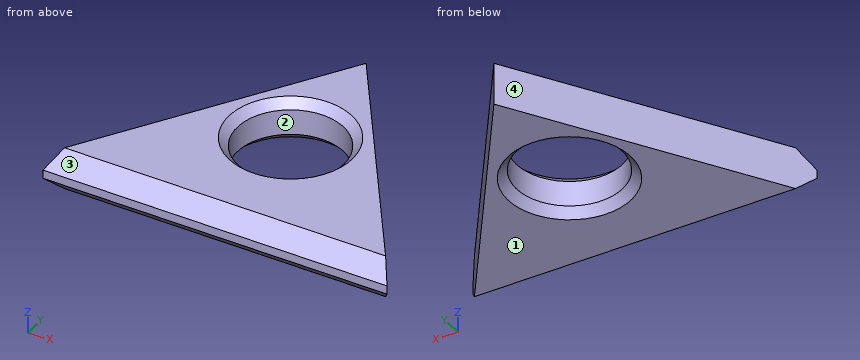
from build123d import *

# Parameters (mm, degrees)
F0_R     = 15.875
F1_DEPTH = 12.7
F2_SIZE  = 5.08
F3_SIZE  = 2.54


with BuildPart() as f1:
    # F0 (on Top) → F1 (new body)
    with BuildSketch(Plane.XY):
        Polygon((0, 76.2), (-50.8, 0), (50.8, 0), align=None)
        with Locations((0, 38.1)):
            Circle(F0_R, mode=Mode.SUBTRACT)
    extrude(amount=F1_DEPTH)

    # F2
    f2_edges = [f1.edges().sort_by_distance(p)[0] for p in [
        (0, 0, 12.7),
        (0, 0, 0),
    ]]
    chamfer(f2_edges, length=F2_SIZE)

    # F3
    f3_edges = [f1.edges().sort_by_distance(p)[0] for p in [
        (-15.875, 38.1, 0),
        (-15.875, 38.1, 12.7),
    ]]
    chamfer(f3_edges, length=F3_SIZE)


solid = f1.part
Can you work these out from the model? Positions are in its coordinate system, mm. Face numbers are marked on the shaded views. Give positions to 0.01 mm unless a question says otherwise; leave off trailing zeros. Loops run counter-clockwise (first coordinate to the right, second up) from the corner with the lowest first, then second, coordinate; pieces in that order, holes last. Notation, with made-up numbers: (70.25, 38.25) -> (129.25, 38.25) arc R11 ccw to (129.25, 53.25) -> close; hole circle Ø6 at (22.5, 52). An arc over 180 degrees is marked (long way). Write item = value, one per line.
1) Suppose I cut it at B-B on x = 22. Write out the boundary of the cut face in (y, z), then the cut area to 3 significant figures.
Check result:
outline = (0, 5.08) -> (5.08, 0) -> (43.2, 0) -> (43.2, 12.7) -> (5.08, 12.7) -> (0, 7.62) -> close
area = 523 mm2
2) Suppose I cut it at D-D on y = 11. Write out the boundary of the cut face in (x, z).
Check result:
outline = (-43.47, 0) -> (43.47, 0) -> (43.47, 12.7) -> (-43.47, 12.7) -> close
3) I need wall thicknesses on L1, parallel to X at y = 29.5, z = 7; L2, parallel to Y at x = 8, z = 2.5; L3, parallel to Y at x = -9, z = 5.75. Which ranges of each line are inside material? Lowest first, please. Write a range as from..to.
Check result:
L1 = -31.13..-13.34, 13.34..31.13
L2 = 2.58..24.34, 51.86..64.2
L3 = 0..25.02, 51.18..62.7
4) Suppose I cut it at A-A on y = 38.1. Write out the boundary of the cut face in (x, z) (3 decimals), then the cut area to 3 significant figures.
Check result:
outline = (-25.4, 0) -> (-18.415, 0) -> (-15.875, 2.54) -> (-15.875, 10.16) -> (-18.415, 12.7) -> (-25.4, 12.7) -> close; (15.875, 2.54) -> (18.415, 0) -> (25.4, 0) -> (25.4, 12.7) -> (18.415, 12.7) -> (15.875, 10.16) -> close
area = 229 mm2
5) Suppose I cut it at C-C on z = 11.5. Write out the boundary of the cut face in (x, y) (3 decimals).
Check result:
outline = (-48.213, 3.88) -> (48.213, 3.88) -> (0, 76.2) -> close; hole circle Ø34.43 at (0, 38.1)
6) Thinking about a two-plate mould opening in Y: for the marked faces 1, 2, 3 and 4, which applies, released by +Y, released by -Y, zero draft, split by the parting line, or undercut?
Check result:
face_1 = zero draft
face_2 = undercut
face_3 = released by -Y
face_4 = released by +Y
7) Will these pins go through, and if not, where does the flat tip stop? pin 1 (4 mm diameter, centred on x = -22, z = 10, fed in from +Y); pin 2 (2 mm diameter, centred on x = 27.5, z = 6.5, fed in from +Y); pin 3 (3 mm diameter, centred on x = -16.5, y = 35, fed in from -Z); pin 4 (4 mm diameter, centred on x = -13, y = 41, fed in from +Z).
Check result:
pin_1 = 46.2
pin_2 = 36.45
pin_3 = 0.13
pin_4 = through
